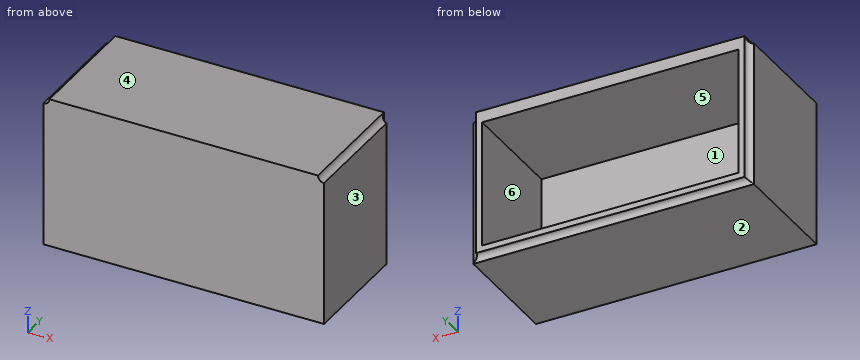
```python
from build123d import *

# Parameters (mm, degrees)
SKETCH_1_W        = 231.607772504
SKETCH_1_H        = 124.691769169
EXTRUDE_1_DEPTH   = 50
SHELL_1_T         = -10
SWEEP_1_PROFILE_R = 5


with BuildPart() as part:
    # 草图1 → 凸台-拉伸1 (new, symmetric)
    with BuildSketch(Plane(origin=(0, 0, 0), x_dir=(1, 0, 0), z_dir=(0, 1, 0))):
        with Locations((-0.653520803, 3.006195692)):
            Rectangle(SKETCH_1_W, SKETCH_1_H)
    extrude(amount=EXTRUDE_1_DEPTH, both=True)

    # 抽壳1
    shell_1_openings = [part.faces().sort_by_distance(p)[0] for p in [
        (-0.653520803, 50, -3.006195693),
    ]]
    offset(amount=SHELL_1_T, openings=shell_1_openings, kind=Kind.INTERSECTION)

    # 切除-扫描1: sweep along a curve in space
    with BuildLine() as sweep_1_path:
        Line((115.150365449, -50, 59.339688892), (115.150365449, 50, 59.339688892))
        Line((115.150365449, 50, 59.339688892), (115.150365449, 50, -65.352080277))
        Line((115.150365449, 50, -65.352080277), (-116.457407055, 50, -65.352080277))
        Line((-116.457407055, 50, -65.352080277), (-116.457407055, 50, 59.339688892))
        Line((-116.457407055, 50, 59.339688892), (-116.457407055, -50, 59.339688892))
    # 切除-扫描1 profile (on start of the path) → 切除-扫描1 (sweep, cut)
    with BuildSketch(Plane(origin=(115.150365449, -50, 59.339688892), x_dir=(0, 0, 1), z_dir=(0, 1, 0))):
        Circle(SWEEP_1_PROFILE_R)
    sweep(path=sweep_1_path.line, transition=Transition.RIGHT, mode=Mode.SUBTRACT)


solid = part.part
```
The model under review builds one solid part; all positions refer to its coordinate system, in mm. Face numbers are marked on the shaded views. A direction names the side the tool comes from. Round coordinates to 2 decimals unless told otherwise and drop trailing zeros. Loops run counter-clockwise (first coordinate to the right, second up) from the corner with the lowest first, then second, coordinate; pieces in that order, holes last. Notation, with made-up numbers: (-13, 35) -> (-8, 35) arc R24 ccw to (-8, 69) -> close; hole circle Ø4 at (8.5, 34.5). An arc over 180 degrees is marked (long way). Answer in a Markdown table with one row per item.
1) Consider section A-A, the plane y = -12.5. Write out the cut boundary in (x, z).
Taken from the geometry:
| item | result |
|---|---|
| outline | (-116.46, -65.35) -> (115.15, -65.35) -> (115.15, 54.34) arc R5 cw to (110.15, 59.34) -> (-111.46, 59.34) arc R5 cw to (-116.46, 54.34) -> close; hole (-106.46, -55.35) -> (105.15, -55.35) -> (105.15, 49.34) -> (-106.46, 49.34) -> close |
2) Consider section C-C, the plane z = 0.5. Write out the cut boundary in (x, y), plus the area to 3 significant figures.
Taken from the geometry:
| item | result |
|---|---|
| outline | (-116.46, -50) -> (115.15, -50) -> (115.15, 45) arc R5 cw to (110.15, 50) -> (105.15, 50) -> (105.15, -40) -> (-106.46, -40) -> (-106.46, 50) -> (-111.46, 50) arc R5 cw to (-116.46, 45) -> close |
| area | 4,080 mm² |
3) Draft analysis for pull direction Z (two halves, no side actions). For the marked faces 3, 4, 5 and 6, state which applies: pulls with the +Z half, pulls with the -Z half, needs draft (parallel to the pull), parting line crosses it, or undercut.
Taken from the geometry:
| item | result |
|---|---|
| face 3 | needs draft |
| face 4 | pulls with the +Z half |
| face 5 | undercut |
| face 6 | undercut |
4) For pin 1 Ø4 at (x, z) = (-70.5, 4) entering from +Y, flat-tipped, find the tip position at first contact; note if it passes through.
Taken from the geometry:
| item | result |
|---|---|
| pin 1 | stops at y = -40 |
5) Wall thickness on line 1 along Z through (x, y) = (9.5, -13); line 2 along X through (y, z) = (5, 45); line 3 along Y through (x, z) = (-56, -40): over which ranges is each line inside the solid? List them lowest first.
Taken from the geometry:
| item | result |
|---|---|
| line 1 | z = -65.35 to -55.35, 49.34 to 59.34 |
| line 2 | x = -116.46 to -106.46, 105.15 to 115.15 |
| line 3 | y = -50 to -40 |
6) Tool access review of the marked faces 1 and 2: name each direction out of +Z, -Z, +X, -X, +Y, -Y from which nothing blocks a thin tool from reaching the whole face with its end or side.
Taken from the geometry:
| item | result |
|---|---|
| face 1 | +Y |
| face 2 | -Z, +X, -X, +Y, -Y |
7) Consider section B-B, the plane x = -61. Write out the cut boundary in (y, z), plus the area to 3 significant figures.
Taken from the geometry:
| item | result |
|---|---|
| outline | (-50, -65.35) -> (45, -65.35) arc R5 cw to (50, -60.35) -> (50, -55.35) -> (-40, -55.35) -> (-40, 49.34) -> (50, 49.34) -> (50, 59.34) -> (-50, 59.34) -> close |
| area | 3,030 mm² |
